Autodesk Inventor part; units mm, degrees
ref_plane "YZ Plane" through (0, 0, 0) normal (1, 0, 0) x (0, 1, 0)
ref_plane "XZ Plane" through (0, 0, 0) normal (0, 1, 0) x (-1, 0, 0)
ref_plane "XY Plane" through (0, 0, 0) normal (0, 0, 1) x (1, 0, 0)
sketch "Sketch1" plane through (0, 0, 0) normal (0, 0, 1) x (1, 0, 0)
  circle A0 centre (0, 0) radius 31.9
  dimension "d0" = 63.8
extrude "Extrusion1" add sketch "Sketch1" against normal blind 1.25
sketch "Sketch2" plane through (0, 0, 0) normal (0, 0, 1) x (1, 0, 0)
  point P0 (0, 0)
  point P1 (-19, -18)
  dimension "d3" = 19
  dimension "d4" = 18
hole "Hole1" at (-19, -18, 0) direction (0, 0, -1) diameter 2 end through all
sketch "Sketch3" plane through (0, 0, 0) normal (0, 0, 1) x (1, 0, 0)
  point P0 (0, 0)
  point P1 (-17.9556, 21)
  point P2 (0, 26.4)
  dimension "d12" = 26.4
  dimension "d101" = 18.75
  dimension "d102" = 21
hole "Hole2" at (-17.9556, 21, 0) at (0, 26.4, 0) direction (0, 0, -1) diameter 2 end through all
sketch "Sketch4" plane through (0, 0, 0) normal (0, 0, 1) x (1, 0, 0)
  point P0 (0, 0)
  point P1 (-12.7, -11.1)
  point P2 (13, -15)
  dimension "d22" = 15
  dimension "d23" = 11.1
  dimension "d24" = 12.7
  dimension "d25" = 13
hole "Hole3" at (-12.7, -11.1, 0) at (13, -15, 0) direction (0, 0, -1) diameter 2.6 end through all
sketch "Sketch5" plane through (0, 0, 0) normal (0, 0, 1) x (1, 0, 0)
  line L0 (-18, 0) -> (18, 0) construction
  point P0 (0, 0)
  point P1 (0, 0)
  dimension "d33" = 36
hole "Hole4" at (18, 0, 0) at (-18, 0, 0) direction (0, 0, -1) diameter 2.8 end through all
sketch "Sketch6" plane through (0, 0, 0) normal (0, 0, 1) x (1, 0, 0)
  point P0 (0, 0)
  point P1 (24, -13.9)
  point P2 (-24, -13.9)
  point P3 (4, 27.5)
  dimension "d41" = 24
  dimension "d42" = 13.9
  dimension "d59" = 4
  dimension "d61" = 24
  dimension "d62" = 13.9
  dimension "d63" = 27.5
hole "Hole5" at (24, -13.9, 0) at (4, 27.5, 0) at (-24, -13.9, 0) direction (0, 0, -1) diameter 3 end through all
sketch "Sketch7" plane through (0, 0, 0) normal (0, 0, 1) x (1, 0, 0)
  point P0 (0, 0)
  point P1 (25.3, 12.7)
  dimension "d50" = 12.7
  dimension "d51" = 25.3
hole "Hole6" at (25.3, 12.7, 0) direction (0, 0, -1) diameter 3.2 end through all
sketch "Sketch8" plane through (0, 0, 0) normal (0, 0, 1) x (1, 0, 0)
  point P0 (0, 0)
  point P1 (0, -15)
  dimension "d64" = 15
hole "Hole7" at (0, -15, 0) direction (0, 0, -1) diameter 4.3 end through all
sketch "Sketch10" plane through (0, 0, 0) normal (0, 0, 1) x (1, 0, 0)
  point P0 (0, 0)
  point P1 (0, 3)
  dimension "d81" = 3
hole "Hole9" at (0, 3, 0) direction (0, 0, -1) diameter 10 end through all
sketch "Sketch11" plane through (0, 0, 0) normal (0, 0, 1) x (1, 0, 0)
  point P0 (0, 0)
  point P1 (0, 0)
  point P2 (28, -5)
  point P3 (28, 5)
  dimension "d91" = 28
  dimension "d92" = 5
  dimension "d93" = 5
hole "Hole10" at (28, -5, 0) at (28, 5, 0) direction (0, 0, -1) diameter 3 end through all
sketch "Sketch12" plane through (0, 0, -1.25) normal (0, 0, -1) x (-1, 0, 0)
  circle A0 centre (0, 0) radius 31.875
  line L0 (0, 0) -> (0, -24.3) construction
  circle A1 centre (0, -24.3) radius 4.25
  point P0 (-3.6509, -26.4756)
  point P1 (3.6509, -26.4756)
  point P2 (-3.6509, -22.1244)
  point P3 (3.6509, -22.1244)
  dimension "d103" = 24.3
  dimension "d104" = 8.5
  dimension "d105" = 63.75
extrude "Extrusion2" cut sketch "Sketch12" against normal through all contours A1
properties part number "403-01" material "Aluminum-6061"
Can you work these out from the model? Positions are in its coordinate system, mm. Round coordinates to 2 decimals unless told otherwise and drop trailing zeros. Write each loop counter-clockwise with the first axis right and the second up, starting at its lowest first coordinate (ties: lowest second). Pieces come first, ordered by that corner, then holes. Notation, with made-up numbers: (-2.5, -4.75) -> (8.5, -4.75) arc R13 cw to (8.5, 15.25) -> close; hole circle Ø7 at (-31.75, -18). An arc over 180 degrees is marked (long way). Use one line per item in the form item = value. Start each with the question number.
Q1. Imagine slicing it at D-D (x = 0). Please give me the cut outline in (y, z).
Q2. I'm going to push a flat-ended pin straight in: P1, Ø2, axis at x = -12.7, y = -11.1, coming from the +Z side (1 decimal). Where does the tip first touch, or does it pass through?
Q3. Imagine slicing it at B-B (x = -12.7). Please give me the cut outline in (y, z), then the cut area to 3 significant figures.
Q4. If I drill on probe 1 along Y at (x, z) = (0, -0.8); probe 2 along Y at (x, z) = (28, -0.9); probe 3 along Y at (x, z) = (25.3, -1), over which ranges is the centre line in solid material (lowest first)? Write a range as [from, to].
Q5. We'd pull the mould along Y, two halves only. Please class faces 1 (the face through (30.427, 9.582, -0.616)), 2 (the face through (7, 0, 0)), 3 (the face through (0, 27.4, -0.6)): +Y half, -Y half, draft (parallel to the pull), parting line (faces both ways), or undercut.
Q6. Imagine slicing it at C-C (z = -0.8). Count the separate pieces of the cut face and the enclosed holes in it, then the cut area to 3 significant figures.
Q7. Imagine slicing it at A-A (y = 0). Please give me the cut outline in (x, z), then the cut area to 4 significant figures.
Worked out:
q1.outline = (-31.9, -1.25) -> (-28.55, -1.25) -> (-28.55, 0) -> (-31.9, 0) -> close; (-20.05, -1.25) -> (-17.15, -1.25) -> (-17.15, 0) -> (-20.05, 0) -> close; (-12.85, -1.25) -> (-2, -1.25) -> (-2, 0) -> (-12.85, 0) -> close; (8, -1.25) -> (25.4, -1.25) -> (25.4, 0) -> (8, 0) -> close; (27.4, -1.25) -> (31.9, -1.25) -> (31.9, 0) -> (27.4, 0) -> close
q2.P1 = through
q3.outline = (-29.26, -1.25) -> (-12.4, -1.25) -> (-12.4, 0) -> (-29.26, 0) -> close; (-9.8, -1.25) -> (29.26, -1.25) -> (29.26, 0) -> (-9.8, 0) -> close
q3.area = 69.9 mm^2
q4.probe_1 = [-31.9, -28.55], [-20.05, -17.15], [-12.85, -2], [8, 25.4], [27.4, 31.9]
q4.probe_2 = [-15.28, -6.5], [-3.5, 3.5], [6.5, 15.28]
q4.probe_3 = [-19.43, -14.65], [-13.15, 11.1], [14.3, 19.43]
q5.face_1 = parting line
q5.face_2 = draft
q5.face_3 = undercut
q6.separate_pieces = 1
q6.enclosed_holes = 16
q6.area = 2,970 mm^2
q7.outline = (-31.9, -1.25) -> (-19.4, -1.25) -> (-19.4, 0) -> (-31.9, 0) -> close; (-16.6, -1.25) -> (-4, -1.25) -> (-4, 0) -> (-16.6, 0) -> close; (4, -1.25) -> (16.6, -1.25) -> (16.6, 0) -> (4, 0) -> close; (19.4, -1.25) -> (31.9, -1.25) -> (31.9, 0) -> (19.4, 0) -> close
q7.area = 62.75 mm^2
